from build123d import *

# Parameters (mm, degrees)
BASIS_BLECH1_DEPTH             = 1
KANTE_LASCHE1_STRIP_W          = 5.4732
KANTE_LASCHE1_STRIP_H          = 1
KANTE_LASCHE1_STRIP_CUT_DEPTH  = 31.657436361
KANTE_LASCHE1_RELIEF_W         = 5.9732
KANTE_LASCHE1_RELIEF_H         = 0.5
KANTE_LASCHE1_RELIEF_CUT_DEPTH = 1
KANTE_LASCHE1_DEPTH            = 31.657436361
KANTE_LASCHE2_STRIP_CUT_DEPTH  = 10.2634
KANTE_LASCHE2_DEPTH            = 10.2634
VERRUNDUNG1_R                  = 0.5


# Sheet-metal steps are written as plain solids
with BuildPart() as part:
    # Skizze1 → Basis-Blech1 (new body)
    with BuildSketch(Plane.XY):
        with BuildLine():
            Line((-42, -8.5), (-42, -16.5))
            ThreePointArc((-42, -16.5), (-41.414213562, -17.914213562), (-40, -18.5))
            Line((-40, -18.5), (-22, -18.5))
            ThreePointArc((-22, -18.5), (-18.464466094, -17.035533906), (-17, -13.5))
            Line((-17, -13.5), (-17, -2.5))
            Line((-17, -2.5), (-28.342563639, -0.5))
            Line((-28.342563639, -0.5), (-60, -0.5))
            Line((-60, -0.5), (-60, -6.5))
            ThreePointArc((-60, -6.5), (-59.414213562, -7.914213562), (-58, -8.5))
            Line((-58, -8.5), (-42, -8.5))
        make_face()
        with BuildLine():
            Line((-29.75, -7.5), (-29.75, -13.5))
            ThreePointArc((-29.75, -13.5), (-32, -15.75), (-34.25, -13.5))
            Line((-34.25, -13.5), (-34.25, -7.5))
            ThreePointArc((-34.25, -7.5), (-32, -5.25), (-29.75, -7.5))
        make_face(mode=Mode.SUBTRACT)
    extrude(amount=BASIS_BLECH1_DEPTH)

    # Kante-Lasche1 strip (across the edge) → Kante-Lasche1 strip cut (cut)
    with BuildSketch(Plane(origin=(-28.342563639, -0.5, 1), x_dir=(0, -1, 0), z_dir=(-1, 0, 0))):
        with Locations((-1, -0.5)):
            Rectangle(KANTE_LASCHE1_STRIP_W, KANTE_LASCHE1_STRIP_H)
    extrude(amount=KANTE_LASCHE1_STRIP_CUT_DEPTH, mode=Mode.SUBTRACT)

    # Kante-Lasche1 relief (on the sheet) → Kante-Lasche1 relief cut (cut)
    with BuildSketch(Plane(origin=(-28.342563639, -2.2366, 1), x_dir=(0, -1, 0), z_dir=(0, 0, 1))):
        with Locations((-2.4866, 0.25)):
            Rectangle(KANTE_LASCHE1_RELIEF_W, KANTE_LASCHE1_RELIEF_H)
    extrude(amount=-KANTE_LASCHE1_RELIEF_CUT_DEPTH, mode=Mode.SUBTRACT)

    # Kante-Lasche1 section (across the edge) → Kante-Lasche1 (add)
    with BuildSketch(Plane(origin=(-28.342563639, -0.5, 1), x_dir=(0, -1, 0), z_dir=(-1, 0, 0))):
        with BuildLine():
            Line((0, 0.7366), (0, 11))
            Line((0, 11), (1, 11))
            Line((1, 11), (1, 0.7366))
            ThreePointArc((1, 0.7366), (1.215745145, 0.215745145), (1.7366, 0))
            Line((1.7366, 0), (1.7366, -1))
            ThreePointArc((1.7366, -1), (0.508638364, -0.491361636), (0, 0.7366))
        make_face()
    extrude(amount=KANTE_LASCHE1_DEPTH)

    # Kante-Lasche2 strip (across the edge) → Kante-Lasche2 strip cut (cut)
    with BuildSketch(Plane(origin=(-28.342563639, -1.5, 1.7366), x_dir=(-0.1736481776669236, -0.9848077530122092, 3.3156835934820577e-15), z_dir=(0, 0, 1))):
        Polygon((-1.92402835, 5.152936518), (-0.973617144, -0.237113276), (0.011190609, -0.063465098), (-0.939220597, 5.326584696), align=None)
    extrude(amount=KANTE_LASCHE2_STRIP_CUT_DEPTH, mode=Mode.SUBTRACT)

    # Kante-Lasche2 section (across the edge) → Kante-Lasche2 (add)
    with BuildSketch(Plane(origin=(-28.342563639, -1.5, 1.7366), x_dir=(-0.1736481776669236, -0.9848077530122092, 3.3156835934820577e-15), z_dir=(0, 0, 1))):
        with BuildLine():
            Line((-1, 0.06444415), (-1, 11.412511336))
            Line((-1, 11.412511336), (0, 11.412511336))
            Line((0, 11.412511336), (0, 0.06444415))
            ThreePointArc((0, 0.06444415), (0.002802985, 0.000245229), (0.011190609, -0.063465098))
            Line((0.011190609, -0.063465098), (-0.973617144, -0.237113276))
            ThreePointArc((-0.973617144, -0.237113276), (-0.993391713, -0.086910513), (-1, 0.06444415))
        make_face()
    extrude(amount=KANTE_LASCHE2_DEPTH)

    # Verrundung1
    verrundung1_edges = [part.edges().sort_by_distance(p)[0] for p in [
        (-17, -2.5, 0.5),
        (-27.842563639, -0.58816349, 0.5),
    ]]
    fillet(verrundung1_edges, radius=VERRUNDUNG1_R)


solid = part.part
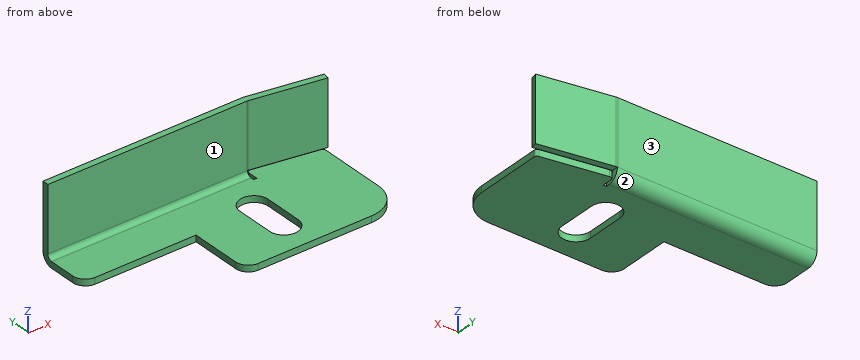
Work out the finished part from the listing and answer in its coordinate system (mm). Face numbers are marked on the shaded views. A direction names the side the tool comes from. Coordinates: 2 decimals unless noted, no trailing zeros. Loops run counter-clockwise (first coordinate to the right, second up) from the corner with the lowest first, then second, coordinate; pieces in that order, holes last. Notation, with made-up numbers: M 20.5,40.5 L 33.5,40.5 A19 cw 33.5,46.5 Z; hole C 15,-30 d10. An arc over 180 degrees is marked long. Answer in a Markdown table with one row per item. Add a question column.
1. Find section C-C, the plane z = 4. Write down the section's boundary in (x, y).
2. Consider L1, parallel to Z at x = -23, y = -11; L2, parallel to Y at x = -49, z = 11.5; L3, parallel to Y at x = -24.5, z = 0.5. Determine where each line is inside the solid, lowest interval first.
3. Find section B-B, the plane x = -32. Write down the section's boundary in (y, z), then the cut area to 3 significant figures.
4. A tool of negligible diameter and unlimited length cuts with its end or side. For the marked faces 1, 2 and 3, from which of +Z, -Z, +X, -X, +Y, -Y can it reach the whole face along a straight path? Write none if from no direction.
5. Find section D-D, the plane x = -44. Write down the section's boundary in (y, z), then the cut area to 3 significant figures.
6. Flat-ended cylindrical pins translate along their axes: P1, Ø0.8, axis at y = -11.5, z = 0.5, coming from the -X side; P2, Ø1.1, axis at y = -10.5, z = 0.5, coming from the +X side; P3, Ø3, axis at x = -50.5, z = 7.5, coming from the -Y side. Find the tip coordinate at first contact, or state that the pin passes through.
7. Find section A-A, the plane y = -11.75. Write down the section's boundary in (x, z).
Reported:
| question | item | result |
|---|---|---|
| 1 | outline | M -60,-1.5 L -28.41,-1.5 A0.74 cw -28.28,-1.51 L -17.1,-3.48 L -16.93,-2.5 L -28.11,-0.53 A1.74 ccw -28.41,-0.5 L -60,-0.5 Z |
| 2 | L1 | z = 0 to 1 |
| 2 | L2 | y = -1.5 to -0.5 |
| 2 | L3 | y = -18.5 to -1.18 |
| 3 | outline | M -18.5,0 L -15.75,0 L -15.75,1 L -18.5,1 Z; M -5.25,0 L -2.24,0 A1.74 ccw -0.5,1.74 L -0.5,12 L -1.5,12 L -1.5,1.74 A0.74 cw -2.24,1 L -5.25,1 Z |
| 3 | area | 18.0 mm^2 |
| 4 | face 1 | +Z, -X, -Y |
| 4 | face 2 | -Z, -X, +Y |
| 4 | face 3 | +Z, -Z, +X, -X, +Y |
| 5 | outline | M -8.5,0 L -2.24,0 A1.74 ccw -0.5,1.74 L -0.5,12 L -1.5,12 L -1.5,1.74 A0.74 cw -2.24,1 L -8.5,1 Z |
| 5 | area | 18.5 mm^2 |
| 6 | P1 | stops at x = -42 |
| 6 | P2 | stops at x = -17 |
| 6 | P3 | stops at y = -1.5 |
| 7 | outline | M -42,0 L -34.25,0 L -34.25,1 L -42,1 Z; M -29.75,0 L -17,0 L -17,1 L -29.75,1 Z |
